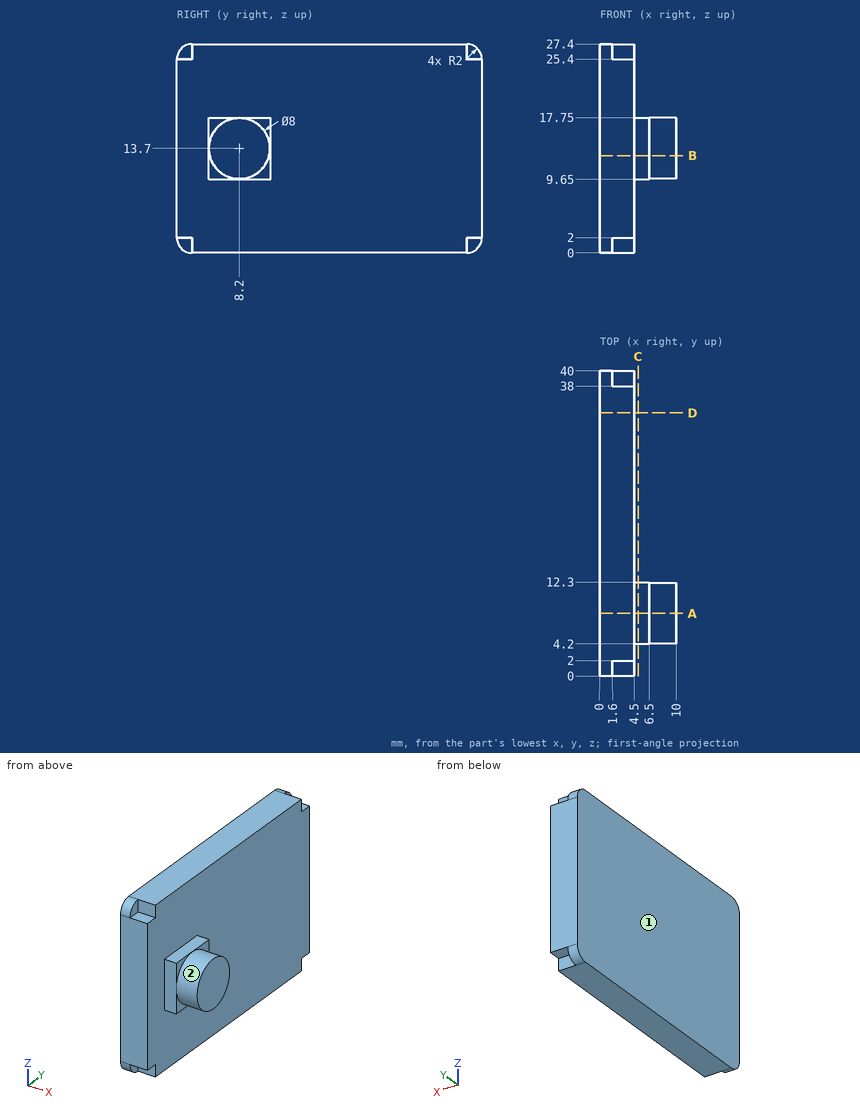
Verification items for this drawing (mm, ordinates from the low corner). A direction names the side the tool comes from. Round coordinates to 2 decimals unless told otherwise and drop trailing zeros. Loops run counter-clockwise (first coordinate to the right, second up) from the corner with the lowest first, then second, coordinate; pieces in that order, holes last. Notation, with made-up numbers: (68.5, -8.5) - (88.5, -8.5) arc R23 ccw to (88.5, 9.5) - close; hole circle Ø11 at (34, 85.25). An arc over 180 degrees is marked (long way). Write item = value, one per line.
Q1. Depth check by flat-ended pin: pin 1 (5 mm diameter, centred on y = 8.5, z = 8, fed in from +X); pin 2 (0.6 mm diameter, centred on x = 2.5, z = 1.5, fed in from +Y); pin 3 (1.6 mm diameter, centred on y = 39, z = 26.5, fed in from +X); pin 4 (1 mm diameter, centred on y = 12, z = 8, fed in from +X). Enter the tip coordinate at first touch or a pass-through.
Here are the results:
pin_1 = 10
pin_2 = 38
pin_3 = 1.6
pin_4 = 4.5
Q2. Sectioned sample at B-B on z = 12.75. Record the boundary of the cut face in (x, y).
Here are the results:
outline = (0, 0) - (4.5, 0) - (4.5, 4.2) - (6.5, 4.2) - (6.5, 4.31) - (10, 4.31) - (10, 12.09) - (6.5, 12.09) - (6.5, 12.3) - (4.5, 12.3) - (4.5, 40) - (0, 40) - close
Q3. Sectioned sample at C-C on x = 5. Record the boundary of the cut face in (y, z), plus the area to 3 significant figures.
Here are the results:
outline = (4.2, 9.65) - (12.3, 9.65) - (12.3, 17.75) - (4.2, 17.75) - close
area = 65.6 mm^2
Q4. Sectioned sample at D-D on y = 34.5. Record the boundary of the cut face in (x, z), plus the area to 3 significant figures.
Here are the results:
outline = (0, 0) - (4.5, 0) - (4.5, 27.4) - (0, 27.4) - close
area = 123 mm^2
Q5. Sectioned sample at A-A on y = 8.2. Record the boundary of the cut face in (x, z).
Here are the results:
outline = (0, 0) - (4.5, 0) - (4.5, 9.65) - (6.5, 9.65) - (6.5, 9.7) - (10, 9.7) - (10, 17.7) - (6.5, 17.7) - (6.5, 17.75) - (4.5, 17.75) - (4.5, 27.4) - (0, 27.4) - close
Q6. Tool access check on the marked faces 1 and 2. Record the directions out of +Z, -Z, +X, -X, +Y, -Y that give a thin tool (end or side, any length) a straight path to the whole face; none if there is none.
Here are the results:
face_1 = +Z, -Z, -X, +Y, -Y
face_2 = +X
Q7. Material ranges on L1, parallel to X at y = 30, z = 19.25; L2, parallel to Y at x = 5.75, z = 11.25; L3, parallel to Z at x = 5, y = 10, recorded low to high.
Here are the results:
L1 = 0 to 4.5
L2 = 4.2 to 12.3
L3 = 9.65 to 17.75
